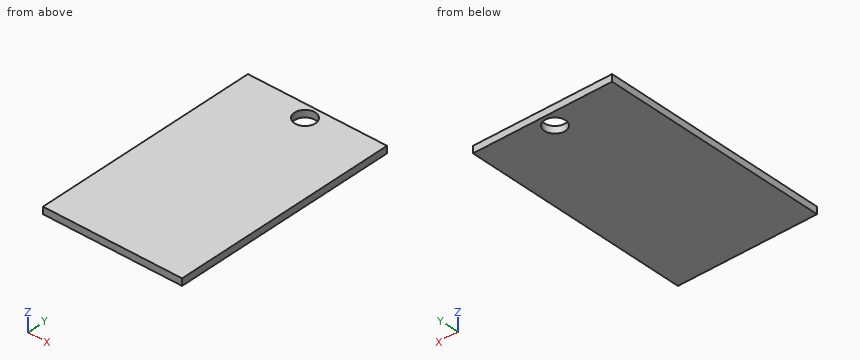
Autodesk Inventor part; units mm, degrees
ref_plane "YZ Plane" through (0, 0, 0) normal (1, 0, 0) x (0, 1, 0)
ref_plane "XZ Plane" through (0, 0, 0) normal (0, 1, 0) x (-1, 0, 0)
ref_plane "XY Plane" through (0, 0, 0) normal (0, 0, 1) x (1, 0, 0)
sketch "Sketch1" plane through (0, 0, 0) normal (0, 0, 1) x (1, 0, 0)
  line L0 (-10, -16.5) -> (10, -16.5)
  line L1 (10, -16.5) -> (10, 16.5)
  line L2 (10, 16.5) -> (-10, 16.5)
  line L3 (-10, 16.5) -> (-10, -16.5)
  line L4 (-10, -16.5) -> (10, 16.5) construction
  line L5 (10, -16.5) -> (-10, 16.5) construction
  line L6 (0, 16.5) -> (0, -16.5)
  line L7 (-10, 0) -> (10, 0)
  circle A0 centre (0, 14.5) radius 1.5
  line L8 (-10, 14.5) -> (10, 14.5) construction
  line L9 (10, 14.5) -> (-10, 14.5) construction
  point P0 (0, 0)
  point P1 (-8, 14.5)
  point P2 (-4, 14.5)
  point P3 (8, 14.5)
  point P4 (4, 14.5)
  point P5 (7, -3.5)
  dimension "d0" = 20
  dimension "d1" = 33
  dimension "d2" = 3
  dimension "d3" = 2
  dimension "d4" = 2
  dimension "d5" = 6
  dimension "d6" = 2
  dimension "d7" = 20
  dimension "d8" = 3
extrude "Extrusion1" add sketch "Sketch1" against normal blind 1
hole "Hole1" at (0, 14.5, 0) direction (0, 0, -1) diameter 3 end through all
properties part number "ShellyUni"
Can you work these out from the model? Positions are in its coordinate system, mm. Give positions to 0.01 mm unless a question says otherwise; leave off trailing zeros. Loops run counter-clockwise (first coordinate to the right, second up) from the corner with the lowest first, then second, coordinate; pieces in that order, holes last. Notation, with made-up numbers: (-29, 66.25) -> (14, 66.25) arc R12 cw to (14, 84.25) -> close; hole circle Ø4 at (-11, 33). An arc over 180 degrees is marked (long way). Use one line per item in the form item = value.
1) If we section it at A-A (x = 0): Please give me the cut outline in (y, z), plus the area to 3 significant figures.
Answers:
outline = (-16.5, -1) -> (13, -1) -> (13, 0) -> (-16.5, 0) -> close; (16, -1) -> (16.5, -1) -> (16.5, 0) -> (16, 0) -> close
area = 30.0 mm²
2) If we section it at B-B (y = 14.5): Please give me the cut outline in (x, z).
Answers:
outline = (-10, -1) -> (-1.5, -1) -> (-1.5, 0) -> (-10, 0) -> close; (1.5, -1) -> (10, -1) -> (10, 0) -> (1.5, 0) -> close
3) I need wall thicknesses on line 1 along X through (y, z) = (14.5, -0.7); line 2 along Y through (x, z) = (0, -0.45); line 3 along Y through (x, z) = (0.75, -0.65). Which ranges of each line are inside material? Lowest first, please.
Answers:
line_1 = -10 to -1.5, 1.5 to 10
line_2 = -16.5 to 13, 16 to 16.5
line_3 = -16.5 to 13.2, 15.8 to 16.5
